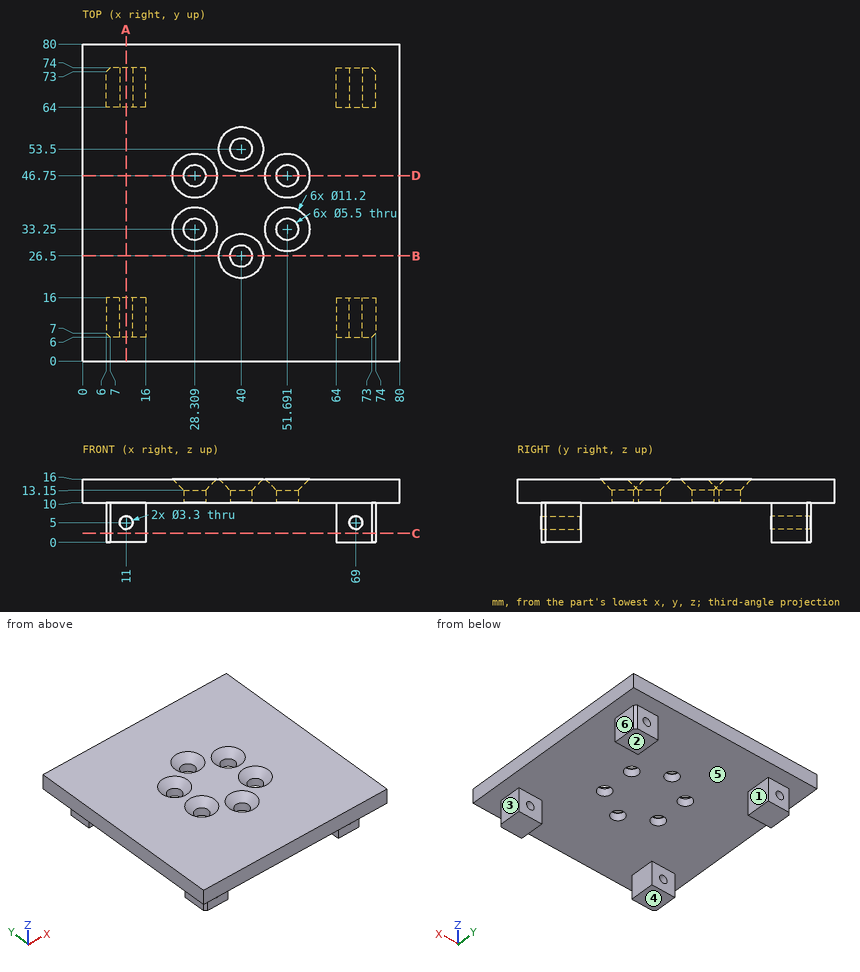
Study the drawing (mm; zero at the part's minimum x, y, z) and answer. A direction names the side the tool comes from. Coordinates: 2 decimals unless noted, no trailing zeros. Write each loop counter-clockwise with the first axis right and the second up, starting at its lowest first coordinate (ties: lowest second). Pieces come first, ordered by that corner, then holes.
Q1. Find the intervals of material crossed by line 1 along Y through (x, z) = (40, 11.05); line 2 along X through (y, z) = (33.25, 10.8); line 3 along X through (y, z) = (12.5, 2), in increasing order.
Returned:
line 1: y = 0 to 23.75, 29.25 to 50.75, 56.25 to 80
line 2: x = 0 to 25.56, 31.06 to 48.94, 54.44 to 80
line 3: x = 6 to 16, 64 to 74
Q2. Given P1, Ø5, axis at y = 10.5, z = 4, coming from the +X side; P2, Ø8, axis at x = 67.5, z = 3.5, coming from the -Y side; P3, Ø5, axis at y = 12, z = 3, coming from the -X side, each flat-ended and moving along its own axis, determine where each tip first touches the part or whether it passes through.
Returned:
P1: stops at x = 74
P2: stops at y = 6
P3: stops at x = 6
Q3. Section A-A, the plane x = 11 is taken. Write down the section's boundary in (y, z), then the cut area to 3 significant figures.
Returned:
outline: (0, 10) - (6, 10) - (6, 6.65) - (16, 6.65) - (16, 10) - (64, 10) - (64, 6.65) - (74, 6.65) - (74, 10) - (80, 10) - (80, 16) - (0, 16) - close; (6, 0) - (16, 0) - (16, 3.35) - (6, 3.35) - close; (64, 0) - (74, 0) - (74, 3.35) - (64, 3.35) - close
area: 614 mm2
Q4. Section D-D, the plane y = 46.75 is taken. Write down the section's boundary in (x, z).
Returned:
outline: (0, 10) - (25.56, 10) - (25.56, 13.15) - (22.71, 16) - (0, 16) - close; (31.06, 10) - (48.94, 10) - (48.94, 13.15) - (46.09, 16) - (33.91, 16) - (31.06, 13.15) - close; (54.44, 10) - (80, 10) - (80, 16) - (57.29, 16) - (54.44, 13.15) - close
Q5. The mould has two halves that part along X. Classify the marked faces 4, 5 and 6: released by +X, released by -X, zero draft, split by the parting line, or undercut.
Returned:
face 4: zero draft
face 5: undercut
face 6: released by +X
Q6. Section B-B, the plane y = 26.5 is taken. Write down the section's boundary in (x, z).
Returned:
outline: (0, 10) - (37.25, 10) - (37.25, 13.15) - (34.4, 16) - (0, 16) - close; (42.75, 10) - (80, 10) - (80, 16) - (45.6, 16) - (42.75, 13.15) - close
Q7. Which of the six approach directions +Z, -Z, +X, -X, +Y, -Y give full straight-line access (tool end or side, diameter ignored) to the marked faces 1, 2 and 3?
Returned:
face 1: -Z, +Y, -Y
face 2: -Z, +X, -X, +Y, -Y
face 3: -Z, +X, +Y, -Y
Q8. Section C-C, the plane z = 2.25 is taken. Write down the section's boundary in (x, y).
Returned:
outline: (6, 7) - (7, 6) - (16, 6) - (16, 16) - (6, 16) - close; (6, 64) - (16, 64) - (16, 74) - (7, 74) - (6, 73) - close; (64, 6) - (73, 6) - (74, 7) - (74, 16) - (64, 16) - close; (64, 64) - (74, 64) - (74, 73) - (73, 74) - (64, 74) - close
